Study the drawing (mm; zero at the part's minimum x, y, z) and answer. Give positions to 0.01 mm unless a question says otherwise; leave off trailing zeros. Loops run counter-clockwise (first coordinate to the right, second up) from the corner with the lowest first, then second, coordinate; pieces in that order, holes last. Notation, with made-up numbers: M 30,-35.75 L 56,-35.75 A26 cw 56,-4.75 Z; hole C 57,-33 d1. An arc over 180 degrees is marked long. Return JSON: item names as keys, results as strings.
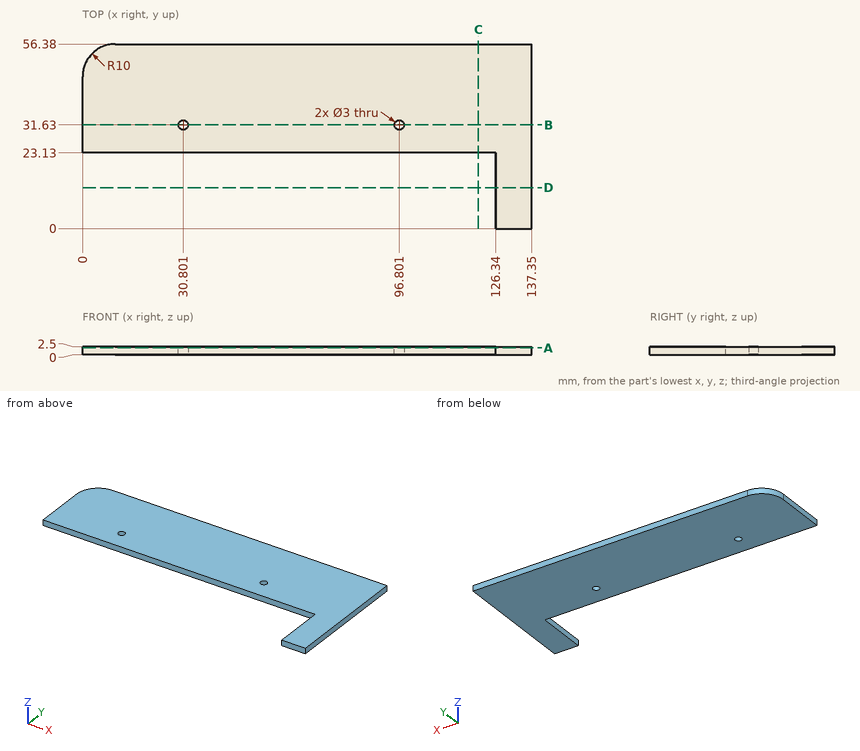
(1) The part is cut by section A-A (z = 2.05). Determine the outline of the cut face in (x, y), and give its area (3 significant figures).
Values follow:
{"outline": "M 0,23.13 L 126.34,23.13 L 126.34,0 L 137.35,0 L 137.35,56.38 L 10,56.38 A10 ccw 0,46.38 Z; hole C 30.8,31.63 d3; hole C 96.8,31.63 d3", "area": "4,790 mm²"}
(2) Straight lines are drawn through the part: line 1 along X through (y, z) = (4, 1.6); line 2 along Y through (x, z) = (43, 1.95); line 3 along Y through (x, z) = (98, 0.3). For each, find the intervals that lie inside material, in ascending order.
Values follow:
{"line 1": "126.34 to 137.35", "line 2": "23.13 to 56.38", "line 3": "23.13 to 30.73, 32.53 to 56.38"}
(3) Given pin 1 (2.5 mm diameter, centred on x = 30.8, y = 31.63, fed in from +Z); pin 2 (1.5 mm diameter, centred on x = 120.5, z = 0.5, fed in from -Y); pin 3 (1.2 mm diameter, centred on y = 6.5, z = 2, fed in from -X); pin 4 (1.5 mm diameter, centred on x = 33.5, y = 29.5, fed in from -Z), each flat-ended and moving along its own axis, determine where each tip first touches the part or whether it passes through.
Values follow:
{"pin 1": "through", "pin 2": "y = 23.13", "pin 3": "x = 126.34", "pin 4": "z = 0"}
(4) The part is cut by section B-B (y = 31.63). Determine the outline of the cut face in (x, z).
Values follow:
{"outline": "M 0,0 L 29.3,0 L 29.3,2.5 L 0,2.5 Z; M 32.3,0 L 95.3,0 L 95.3,2.5 L 32.3,2.5 Z; M 98.3,0 L 137.35,0 L 137.35,2.5 L 98.3,2.5 Z"}
(5) The part is cut by section D-D (y = 12.5). Determine the outline of the cut face in (x, z).
Values follow:
{"outline": "M 126.34,0 L 137.35,0 L 137.35,2.5 L 126.34,2.5 Z"}
(6) The part is cut by section C-C (x = 121). Determine the outline of the cut face in (y, z).
Values follow:
{"outline": "M 23.13,0 L 56.38,0 L 56.38,2.5 L 23.13,2.5 Z"}
